Input: part model. Units: mm. Frame: model coordinates. A direction names the side the tool comes from. Give positions to 0.01 mm unless a question says otherwise; leave off trailing zeros. Write each loop counter-clockwise with the first axis right and the second up, starting at its lowest first coordinate (ties: lowest second). Pieces come first, ordered by that corner, then holes. Notation, with made-up numbers: (-38, -30) - (-16, -30) arc R28 ccw to (-16, 4) - close; hole circle Ø5 at (-32, -38.75). An arc over 180 degrees is marked (long way). Answer as CSV lines item,"result". Start each with the question number.
from build123d import *

# Parameters (mm, degrees)
BOSS_EXTRU_1_DEPTH      = 5
BOSS_EXTRU_2_DEPTH      = 10
ESQUISSE4_R             = 2.8
ENL_V_MAT_EXTRU_1_DEPTH = 9.1
ESQUISSE5_R             = 2.8
ENL_V_MAT_EXTRU_2_DEPTH = 9.1
ESQUISSE6_R             = 2.8
ENL_V_MAT_EXTRU_3_DEPTH = 9.1
BOSS_EXTRU_3_DEPTH      = 8
ESQUISSE8_R             = 2.1
ENL_V_MAT_EXTRU_5_DEPTH = 9.1
ESQUISSE9_R             = 2.1
ENL_V_MAT_EXTRU_6_DEPTH = 14
CONG_2_R                = 5
CONG_1_R                = 2


with BuildPart() as part:
    # Esquisse2 → Boss.-Extru.1 (new body)
    with BuildSketch(Plane(origin=(0, 0, 0), x_dir=(1, 0, 0), z_dir=(0, 1, 0))):
        Polygon((20, 0), (0, 0), (0, -20), (0, -40), (-15, -40), (-15, -15), (-14.241244466, -15), (2.1313405, 13.65202369), (0, 15), (32, 15), (32, 0), align=None)
    extrude(amount=BOSS_EXTRU_1_DEPTH)

    # Esquisse3 → Boss.-Extru.2 (add)
    with BuildSketch(Plane(origin=(0, 5, 0), x_dir=(1, 0, 0), z_dir=(0, 1, 0))):
        Polygon((32, 15), (20, 15), (20, 3), (8.713731996, 3), (8.713731996, 8.738906014), (1.635201562, 12.783780548), (-13.745105527, -14.131756858), (-4, -19.700388588), (-4, -28), (-15, -28), (-15, -40), (0, -40), (0, 0), (32, 0), align=None)
    extrude(amount=BOSS_EXTRU_2_DEPTH)

    # Esquisse4 → Enlèv. mat.-Extru.1 (cut)
    with BuildSketch(Plane(origin=(-4.274168905, 0, -2.442382231), x_dir=(-0.4961389383568338, 0, 0.8682431421244592), z_dir=(-0.8682431421244592, 0, -0.4961389383568338))):
        with Locations((-6.410716958, 10)):
            Circle(ESQUISSE4_R)
        with Locations((13.589283042, 10)):
            Circle(ESQUISSE4_R)
    extrude(amount=-ENL_V_MAT_EXTRU_1_DEPTH, mode=Mode.SUBTRACT)

    # Esquisse5 → Enlèv. mat.-Extru.2 (cut)
    with BuildSketch(Plane.ZY.offset(15)):
        with Locations((34, 10)):
            Circle(ESQUISSE5_R)
    extrude(amount=-ENL_V_MAT_EXTRU_2_DEPTH, mode=Mode.SUBTRACT)

    # Esquisse6 → Enlèv. mat.-Extru.3 (cut)
    with BuildSketch(Plane(origin=(0, 0, -15), x_dir=(-1, 0, 0), z_dir=(0, 0, -1))):
        with Locations((-26, 10)):
            Circle(ESQUISSE6_R)
    extrude(amount=-ENL_V_MAT_EXTRU_3_DEPTH, mode=Mode.SUBTRACT)

    # Esquisse10 → Boss.-Extru.3 (add)
    with BuildSketch(Plane(origin=(0, 15, 0), x_dir=(1, 0, 0), z_dir=(0, 1, 0))):
        Polygon((15, 3), (8.713731996, 3), (5, 3), (5, 0), (15, 0), align=None)
    extrude(amount=BOSS_EXTRU_3_DEPTH)

    # Esquisse8 → Enlèv. mat.-Extru.5 (cut)
    with BuildSketch(Plane.XY):
        with Locations((10, 19)):
            Circle(ESQUISSE8_R)
    extrude(amount=-ENL_V_MAT_EXTRU_5_DEPTH, mode=Mode.SUBTRACT)

    # Esquisse9 → Enlèv. mat.-Extru.6 (cut)
    with BuildSketch(Plane(origin=(0, 5, 0), x_dir=(1, 0, 0), z_dir=(0, 1, 0))):
        with Locations(Location((-10, -22, 0), (0, 0, 270))):
            Circle(ESQUISSE9_R)
        with Locations(Location((14, 10, 0), (0, 0, 270))):
            Circle(ESQUISSE9_R)
    extrude(amount=-ENL_V_MAT_EXTRU_6_DEPTH, mode=Mode.SUBTRACT)

    # Congé2
    cong_2_edges = [part.edges().sort_by_distance(p)[0] for p in [
        (15, 15, -1.5),
        (5, 15, -1.5),
    ]]
    fillet(cong_2_edges, radius=CONG_2_R)

    # Congé1
    cong_1_edges = [part.edges().sort_by_distance(p)[0] for p in [
        (15, 23, -1.5),
        (5, 23, -1.5),
        (32, 7.5, 0),
        (0, 7.5, 40),
        (20, 10, -3),
        (8.713731996, 10, -8.738906014),
        (-4, 10, 19.700388588),
        (-4, 10, 28),
    ]]
    fillet(cong_1_edges, radius=CONG_1_R)


solid = part.part
1) Pull-direction query (X, two-part tool) for faces 4 (the cylindrical face through (2.982, 12.776, -6.099)), 5 (the cylindrical face through (-0.6, 7.6, 39.43)), 6 (the cylindrical face through (8.452, 20.419, -1.479)), 7 (the cylindrical face through (-4.57, 10.07, 27.4)); classes: +X half, -X half, draft (parallel to the pull), parting line (faces both ways), or undercut.
2) Material intervals for line 1 (Y direction, x = -9.75, z = 34); line 2 (Y direction, x = 10, z = -2), sorted ascending. Write a range as from..to.
3) Contact query for flat-ended pins moving along their axis: P1, Ø9.5, axis at x = 7, z = -10.5, coming from the +Y side; P2, Ø4, axis at x = 18.5, y = 3, coming from the +Z side; P3, Ø3.5, axis at x = -10, z = 22, coming from the +Y side; P4, Ø3, axis at y = 9.5, z = -10.5, coming from the -X side. Output: stop coordinate, or through.
4) Cut plane B-B on z = 22. Output: boundary loops of the cut face in (x, y).
5) Cut plane C-C on y = 3. Output: boundary loops of the cut face in (x, z), and give its area (3 significant figures).
6) Cut plane A-A on x = 10. Output: boundary loops of the cut face in (y, z).
7) Cut plane D-D on z = 34. Output: boundary loops of the cut face in (x, y), and give its area (3 significant figures).
8) Reachability of faces 1 (the flat face through (15, 9, 0)), 2 (the flat face through (-10, 10, 28)), 3 (the cylindrical face through (-10.514, 11.892, 31.936)) from +Z, -Z, +X, -X, +Y, -Y: full face, straight path, thin tool, end or side. Return the list, or none.
Numbers:
1,face 4,"undercut"
1,face 5,"+X half"
1,face 6,"undercut"
1,face 7,"-X half"
2,line 1,"y = 0..7.2, 12.8..15"
2,line 2,"y = 0..16.9, 21.1..23"
3,P1,"stops at y = 15"
3,P2,"stops at z = 0"
3,P3,"passes through"
3,P4,"stops at x = -0.05"
4,outline,"(-15, 0) - (-12.1, 0) - (-12.1, 5) - (-15, 5) - close; (-7.9, 0) - (0, 0) - (0, 15) - (-4, 15) - (-4, 5) - (-7.9, 5) - close"
5,outline,"(-15, 15) - (-14.24, 15) - (2.13, -13.65) - (0, -15) - (32, -15) - (32, -2) arc R2 ccw to (30, 0) - (0, 0) - (0, 38) arc R2 ccw to (-2, 40) - (-15, 40) - close; hole circle Ø4.2 at (-10, 22); hole circle Ø4.2 at (14, -10)"
5,area,"998 mm²"
6,outline,"(0, -15) - (5, -15) - (5, -3) - (16.9, -3) - (16.9, 0) - (0, 0) - close; (21.1, -3) - (23, -3) - (23, 0) - (21.1, 0) - close"
7,outline,"(-15, 0) - (0, 0) - (0, 15) - (-15, 15) - (-15, 12.8) - (-5.9, 12.8) - (-5.9, 7.2) - (-15, 7.2) - close"
7,area,"174 mm²"
8,face 1,"+Z, +X, +Y, -Y"
8,face 2,"-X, +Y"
8,face 3,"-X"
